Part model, mm, in its own coordinate system. A direction names the side the tool comes from. Round coordinates to 2 decimals unless told otherwise and drop trailing zeros. Write each loop counter-clockwise with the first axis right and the second up, starting at its lowest first coordinate (ties: lowest second). Pieces come first, ordered by that corner, then holes. Notation, with made-up numbers: (79, -19.75) -> (85, -19.75) arc R16 ccw to (85, -1.75) -> close; hole circle Ø4 at (76.5, 69.25). An arc over 180 degrees is marked (long way). Use CSV: the item, a comma, the result in double quotes. Start each with the question number.
(1) Saw through at A-A (x = 0.15). Give the cut face in (y, z) (3 decimals), plus the area to 3 significant figures.
(2) Drop flat-ended pins along their axis: pin 1 (2 mm diameter, centred on x = 0, z = 1.5, fed in from -Y); pin 2 (0.9 mm diameter, centred on x = 0, y = 48, fed in from -Z) (3 decimals); pin 3 (1.2 mm diameter, centred on x = 1, z = -4, fed in from -Y); pin 4 (0.9 mm diameter, centred on x = 0, y = 30.5, fed in from +Z) (3 decimals). Give the stop position or say it passes through.
(3) Probe line 1 (X direction, y = 43.5, z = 4) (3 decimals); line 2 (Y direction, x = -0.55, z = 3.75); line 3 (Z direction, x = -0.7, y = 40) (3 decimals). List the from-to ranges inside material, lowest first. Write a range as [from, to].
(4) Two-plate mould, pull along X, no slides. Class faces 6 (the flat face through (0, 39, 2.625)), 7 (the flat face through (0, 0, 0)), 8 (the flat face through (-2.625, 30, 0)), 9 (the flat face through (2.625, 30, 0)): released by +X, released by -X, zero draft, split by the parting line, or undercut.
(5) Saw through at C-C (y = 50.5). Give the cut face in (x, z) (3 decimals), plus the area to 3 significant figures.
(6) Which spindle directions (+Z, -Z, +X, -X, +Y, -Y) get a long thin tool onto all of the face, cutting with end or side? Do faces 1 (the flat face through (0, 16, 5)), 2 (the flat face through (0, 6, -5)), 3 (the flat face through (-1.2, 33.1, 6.625)), 4 (the flat face through (0, 3, 2.625)), 5 (the flat face through (0, 39, -2.625)). Say none if no direction does.
(7) Saw through at B-B (z = -3.75). Give the cut face in (x, y) (3 decimals), plus the area to 3 significant figures.
```python
from build123d import *

# Parameters (mm, degrees)
SKETCH1_W           = 5.25
SKETCH1_H           = 5.25
BOSS_EXTRUDE1_DEPTH = 6
SKETCH2_W           = 5.25
SKETCH2_H           = 9.25
BOSS_EXTRUDE2_DEPTH = 55
SKETCH3_W           = 1.75
SKETCH3_H           = 8
CUT_EXTRUDE1_DEPTH  = 45
SKETCH4_W           = 5.25
SKETCH4_H           = 55
BOSS_EXTRUDE3_DEPTH = 4
SKETCH5_W           = 1.75
SKETCH5_H           = 8
CUT_EXTRUDE2_DEPTH  = 45


with BuildPart() as part:
    # Sketch1 → Boss-Extrude1 (new body)
    with BuildSketch(Plane(origin=(0, 0, 0), x_dir=(1, 0, 0), z_dir=(0, 1, 0))):
        Rectangle(SKETCH1_W, SKETCH1_H)
    extrude(amount=BOSS_EXTRUDE1_DEPTH)

    # Sketch2 → Boss-Extrude2 (add)
    with BuildSketch(Plane(origin=(0, 6, 0), x_dir=(1, 0, 0), z_dir=(0, 1, 0))):
        with Locations((0, -2)):
            Rectangle(SKETCH2_W, SKETCH2_H)
    extrude(amount=BOSS_EXTRUDE2_DEPTH)

    # Sketch3 → Cut-Extrude1 (cut)
    with BuildSketch(Plane(origin=(0, 61, 0), x_dir=(1, 0, 0), z_dir=(0, 1, 0))):
        with Locations((0, -6.625)):
            Rectangle(SKETCH3_W, SKETCH3_H)
    extrude(amount=-CUT_EXTRUDE1_DEPTH, mode=Mode.SUBTRACT)

    # Sketch4 → Boss-Extrude3 (add)
    with BuildSketch(Plane(origin=(0, 0, -2.625), x_dir=(-1, 0, 0), z_dir=(0, 0, -1))):
        with Locations((0, 33.5)):
            Rectangle(SKETCH4_W, SKETCH4_H)
    extrude(amount=BOSS_EXTRUDE3_DEPTH)

    # Sketch5 → Cut-Extrude2 (cut)
    with BuildSketch(Plane(origin=(0, 61, 0), x_dir=(1, 0, 0), z_dir=(0, 1, 0))):
        with Locations((0, 6.625)):
            Rectangle(SKETCH5_W, SKETCH5_H)
    extrude(amount=-CUT_EXTRUDE2_DEPTH, mode=Mode.SUBTRACT)


solid = part.part
```
Answers:
1,outline,"(0, -2.625) -> (6, -2.625) -> (6, -6.625) -> (16, -6.625) -> (16, -2.625) -> (61, -2.625) -> (61, 2.625) -> (16, 2.625) -> (16, 6.625) -> (6, 6.625) -> (6, 2.625) -> (0, 2.625) -> close"
1,area,"400 mm²"
2,pin 1,"stops at y = 0"
2,pin 2,"stops at z = -2.625"
2,pin 3,"stops at y = 6"
2,pin 4,"stops at z = 2.625"
3,line 1,"x = [-2.625, -0.875], [0.875, 2.625]"
3,line 2,"y = [6, 16]"
3,line 3,"z = [-2.625, 2.625]"
4,face 6,"undercut"
4,face 7,"zero draft"
4,face 8,"released by -X"
4,face 9,"released by +X"
5,outline,"(-2.625, -6.625) -> (-0.875, -6.625) -> (-0.875, -2.625) -> (0.875, -2.625) -> (0.875, -6.625) -> (2.625, -6.625) -> (2.625, 6.625) -> (0.875, 6.625) -> (0.875, 2.625) -> (-0.875, 2.625) -> (-0.875, 6.625) -> (-2.625, 6.625) -> close"
5,area,"55.6 mm²"
6,face 1,"+Z, +Y"
6,face 2,"-Z, +X, -X, -Y"
6,face 3,"+Z, +X, -X, +Y, -Y"
6,face 4,"+Z, +X, -X, -Y"
6,face 5,"-Z, +Y"
7,outline,"(-2.625, 6) -> (2.625, 6) -> (2.625, 61) -> (0.875, 61) -> (0.875, 16) -> (-0.875, 16) -> (-0.875, 61) -> (-2.625, 61) -> close"
7,area,"210 mm²"
